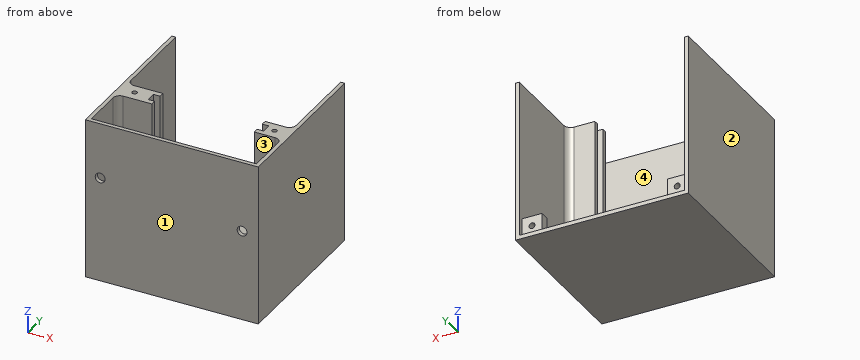
from build123d import *

# Parameters (mm, degrees)
SKETCH1_W           = 52.4
SKETCH1_H           = 49.3
BOSS_EXTRUDE1_DEPTH = 49
CUT_EXTRUDE1_DEPTH  = 47.8
SKETCH3_W           = 6
SKETCH3_H           = 3
BOSS_EXTRUDE2_DEPTH = 6
SKETCH4_R           = 0.75
CUT_EXTRUDE2_DEPTH  = 10
SKETCH5_R           = 1.5
CUT_EXTRUDE3_DEPTH  = 74.491836281
SKETCH6_R           = 0.9
CUT_EXTRUDE4_DEPTH  = 5
FILLET1_R           = 2


with BuildPart() as part:
    # Sketch1 → Boss-Extrude1 (new body)
    with BuildSketch(Plane.XY):
        with Locations((0, 24.65)):
            Rectangle(SKETCH1_W, SKETCH1_H)
    extrude(amount=BOSS_EXTRUDE1_DEPTH)

    # Sketch2 → Cut-Extrude1 (cut)
    with BuildSketch(Plane.XY.offset(49)):
        Polygon((25, 1.2), (25, 15.6), (16.7, 15.6), (16.7, 17.2), (18.7, 17.2), (18.7, 20.2), (16.7, 20.2), (16.7, 21.8), (25, 21.8), (25, 49.3), (-25, 49.3), (-25, 21.8), (-14.3, 21.8), (-14.3, 20.2), (-16.3, 20.2), (-16.3, 17.2), (-14.3, 17.2), (-14.3, 15.6), (-25, 15.6), (-25, 1.2), align=None)
    extrude(amount=-CUT_EXTRUDE1_DEPTH, mode=Mode.SUBTRACT)

    # Sketch3 → Boss-Extrude2 (add)
    with BuildSketch(Plane.XY.offset(1.2)):
        with Locations((-22, 46.2)):
            Rectangle(SKETCH3_W, SKETCH3_H)
        with Locations((22, 46.2)):
            Rectangle(SKETCH3_W, SKETCH3_H)
    extrude(amount=BOSS_EXTRUDE2_DEPTH)

    # Sketch4 → Cut-Extrude2 (cut)
    with BuildSketch(Plane.XY.offset(49)):
        with Locations((-21.2, 18.7)):
            Circle(SKETCH4_R)
        with Locations((21.2, 18.7)):
            Circle(SKETCH4_R)
    extrude(amount=-CUT_EXTRUDE2_DEPTH, mode=Mode.SUBTRACT)

    # Sketch5 → Cut-Extrude3 (cut, through all)
    with BuildSketch(Plane(origin=(0, 1.2, 0), x_dir=(1, 0, 0), z_dir=(0, 1, 0))):
        with Locations(Location((-21.7, -32.1, 0), (0, 0, 270))):
            Circle(SKETCH5_R)
        with Locations(Location((21.3, -27.6, 0), (0, 0, 270))):
            Circle(SKETCH5_R)
    extrude(amount=-CUT_EXTRUDE3_DEPTH, mode=Mode.SUBTRACT)

    # Sketch6 → Cut-Extrude4 (cut)
    with BuildSketch(Plane(origin=(0, 47.7, 0), x_dir=(1, 0, 0), z_dir=(0, 1, 0))):
        with Locations(Location((22, -4.2, 0), (0, 0, 180))):
            Circle(SKETCH6_R)
        with Locations(Location((-22, -4.2, 0), (0, 0, 180))):
            Circle(SKETCH6_R)
    extrude(amount=-CUT_EXTRUDE4_DEPTH, mode=Mode.SUBTRACT)

    # Fillet1
    fillet1_edges = [part.edges().sort_by_distance(p)[0] for p in [
        (-25, 15.6, 25.1),
        (-25, 21.8, 25.1),
        (25, 21.8, 25.1),
        (25, 15.6, 25.1),
        (-25, 44.7, 4.2),
        (25, 44.7, 4.2),
    ]]
    fillet(fillet1_edges, radius=FILLET1_R)


solid = part.part
The listing builds one solid part. Answer for the finished solid, in the listing's coordinates (mm). Face numbers are marked on the shaded views. A direction names the side the tool comes from. Coordinates: 2 decimals unless noted, no trailing zeros. Write each loop counter-clockwise with the first axis right and the second up, starting at its lowest first coordinate (ties: lowest second). Pieces come first, ordered by that corner, then holes. Notation, with made-up numbers: (23, 30.25) - (48, 30.25) arc R20 cw to (48, 49.25) - close; hole circle Ø11 at (64, 73.25). An arc over 180 degrees is marked (long way). Put each result on its own line as item: value.
1. Find the intervals of material crossed by line 1 along Y through (x, z) = (18.5, 39); line 2 along Y through (x, z) = (21.2, 42.5); line 3 along X through (y, z) = (0.95, 32.1), in increasing order. Write a range as from..to.
Answer sheet:
line 1: y = 0..1.2, 15.6..17.2, 20.2..21.8
line 2: y = 0..1.2, 15.6..17.95, 19.45..21.8
line 3: x = -26.2..-23.2, -20.2..26.2
2. The part is cut by section B-B on z = 37. Give the vertices of the cut face in (x, y), plus the area to 3 significant figures.
Answer sheet:
outline: (-26.2, 0) - (26.2, 0) - (26.2, 49.3) - (25, 49.3) - (25, 23.8) arc R2 cw to (23, 21.8) - (16.7, 21.8) - (16.7, 20.2) - (18.7, 20.2) - (18.7, 17.2) - (16.7, 17.2) - (16.7, 15.6) - (23, 15.6) arc R2 cw to (25, 13.6) - (25, 1.2) - (-25, 1.2) - (-25, 13.6) arc R2 cw to (-23, 15.6) - (-14.3, 15.6) - (-14.3, 17.2) - (-16.3, 17.2) - (-16.3, 20.2) - (-14.3, 20.2) - (-14.3, 21.8) - (-23, 21.8) arc R2 cw to (-25, 23.8) - (-25, 49.3) - (-26.2, 49.3) - close
area: 288 mm^2
3. A tool of negligible diameter and unlimited length cuts with its end or side. For the marked faces 4 and 5, from which of +Z, -Z, +X, -X, +Y, -Y can it reach the whole face along a straight path? Write none if from no direction.
Answer sheet:
face 4: +Z
face 5: +Z, -Z, +X, +Y, -Y
4. The part is cut by section C-C on x = 10. Give the vertices of the cut face in (y, z), plus the area to 3 significant figures.
Answer sheet:
outline: (0, 0) - (49.3, 0) - (49.3, 1.2) - (1.2, 1.2) - (1.2, 49) - (0, 49) - close
area: 117 mm^2
5. The part is cut by section A-A on y = 29. Give the vertices of the cut face in (x, z).
Answer sheet:
outline: (-26.2, 0) - (26.2, 0) - (26.2, 49) - (25, 49) - (25, 1.2) - (-25, 1.2) - (-25, 49) - (-26.2, 49) - close
6. Determine the mould class of the marked faces 1, 2 and 3 for opening direction X: pulls with the +X half, pulls with the -X half, needs draft (parallel to the pull), parting line crosses it, or undercut.
Answer sheet:
face 1: needs draft
face 2: pulls with the -X half
face 3: undercut
7. Flat-ended cylindrical pins translate along their axes: pin 1 Ø1.5 at (x, z) = (-9.5, 16.5) entering from +Y; pin 2 Ø1 at (x, z) = (-15, 14) entering from +Y; pin 3 Ø3 at (x, y) = (-16, 29.5) entering from +Z. Find the tip coordinate at first contact, or state that the pin passes through.
Answer sheet:
pin 1: stops at y = 1.2
pin 2: stops at y = 21.8
pin 3: stops at z = 1.2
